from build123d import *

# Parameters (mm, degrees)
SKETCH1_R           = 7
SKETCH1_R_2         = 2.5
BOSS_EXTRUDE1_DEPTH = 6.35


with BuildPart() as part:
    # Sketch1 → Boss-Extrude1 (new, symmetric)
    with BuildSketch(Plane(origin=(0, 0, 0), x_dir=(1, 0, 0), z_dir=(0, 1, 0))):
        with BuildLine():
            Line((20, 0), (0, 0))
            Line((0, 0), (0, 60))
            Line((0, 60), (32, 60))
            ThreePointArc((32, 60), (48.687461624, 46.244784205), (38.370260223, 27.23866171))
            ThreePointArc((38.370260223, 27.23866171), (25.021742974, 16.427196599), (20, 0))
        make_face()
        with Locations(Location((32, 43, 0), (0, 0, 270))):
            Circle(SKETCH1_R, mode=Mode.SUBTRACT)
        with Locations(Location((10, 10, 0), (0, 0, 270))):
            Circle(SKETCH1_R_2, mode=Mode.SUBTRACT)
        with Locations(Location((10, 50, 0), (0, 0, 270))):
            Circle(SKETCH1_R_2, mode=Mode.SUBTRACT)
    extrude(amount=BOSS_EXTRUDE1_DEPTH, both=True)


solid = part.part
Verification items for the finished model (mm, model axes). Coordinates: 2 decimals unless noted, no trailing zeros. Order: outer loops, then holes, each group sorted by start corner. A loop starts at its lowest first (then second) coordinate and runs counter-clockwise, first axis right, second up.
Item 1: Section check B-B, the plane y = 3.75. Enter the section's corners in (x, z).
Filled in:
outline: (0, -60) - (32, -60) arc R17 ccw to (38.37, -27.24) arc R29.38 cw to (20, 0) - (0, 0) - close; hole circle Ø5 at (10, -50); hole circle Ø5 at (10, -10); hole circle Ø14 at (32, -43)
Item 2: Section check D-D, the plane z = -10. Enter the section's corners in (x, y).
Filled in:
outline: (0, -6.35) - (7.5, -6.35) - (7.5, 6.35) - (0, 6.35) - close; (12.5, -6.35) - (21.75, -6.35) - (21.75, 6.35) - (12.5, 6.35) - close
Item 3: Release check for a two-part mould opening along X. For faces 1 (the face through (16, 0, -60)), 2 (the face through (9.04, -0.09, -47.69)), 3 (the face through (25.16, 0.09, -16.63)) record: +X half, -X half, draft (parallel to the pull), parting line (faces both ways), or undercut.
Filled in:
face 1: draft
face 2: undercut
face 3: +X half
Item 4: Depth check by flat-ended pin: pin 1 (1 mm diameter, centred on y = -2.5, z = -49, fed in from +X); pin 2 (12 mm diameter, centred on x = 35, z = -20.5, fed in from -Y); pin 3 (6 mm diameter, centred on y = 5, z = -15, fed in from +X); pin 4 (1.5 mm diameter, centred on x = 31, y = -2, fed in from +Z). Enter the tip coordinate at first touch or a pass-through.
Filled in:
pin 1: stops at x = 48.09
pin 2: stops at y = -6.35
pin 3: stops at x = 26.16
pin 4: stops at z = -22.3
Item 5: Section check A-A, the plane z = -43. Enter the section's corners in (x, y).
Filled in:
outline: (0, -6.35) - (25, -6.35) - (25, 6.35) - (0, 6.35) - close; (39, -6.35) - (49, -6.35) - (49, 6.35) - (39, 6.35) - close
Item 6: Section check C-C, the plane x = 11. Enter the section's corners in (y, z).
Filled in:
outline: (-6.35, -60) - (6.35, -60) - (6.35, -52.29) - (-6.35, -52.29) - close; (-6.35, -47.71) - (6.35, -47.71) - (6.35, -12.29) - (-6.35, -12.29) - close; (-6.35, -7.71) - (6.35, -7.71) - (6.35, 0) - (-6.35, 0) - close
Item 7: Material ranges on L1, parallel to X at y = -4.5, z = -11; L2, parallel to X at y = 2, z = -52; L3, parallel to Z at x = 33, y = 3, recorded low to high.
Filled in:
L1: x = 0 to 7.71, 12.29 to 22.14
L2: x = 0 to 8.5, 11.5 to 46.42
L3: z = -59.97 to -49.93, -36.07 to -24.39
